Could you check a few things on this model? Use its own coordinates, in mm. Face numbers are marked on the shaded views. Give positions to 0.01 mm unless a question says otherwise; leave off trailing zeros. Order: outer loops, then holes, each group sorted by start corner. A loop starts at its lowest first (then second) coordinate and runs counter-clockwise, first axis right, second up. Notation, with made-up numbers: (81.25, 6) -> (130.25, 6) arc R7 ccw to (130.25, 11) -> close; hole circle Ø6 at (-32, 7). An arc over 180 degrees is marked (long way). Use one line per item in the form item = value. Start each with the question number.
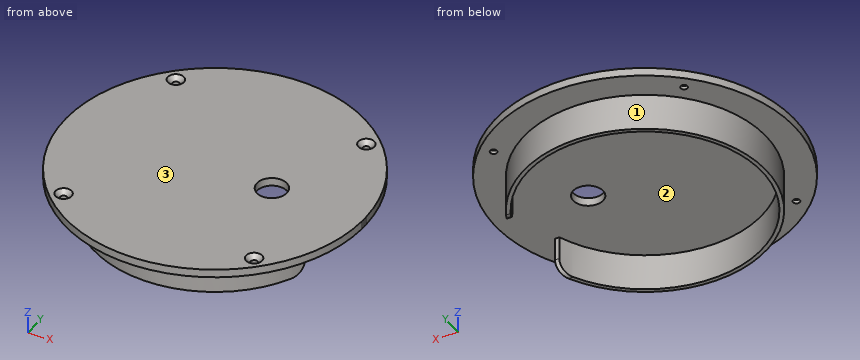
from build123d import *

# Parameters (mm, degrees)
F0_R        = 1.25
F0_R_2      = 5.5
F1_DEPTH    = 3
F3_DEPTH    = 13.4
F4_T1_DEPTH = 26.5968204778
F5_SIZE     = 1.7


# Not quite as in the source:
# - a fillet or chamfer that OpenCascade refuses, or shapes differently, is made with other operations: its cross-section is extruded or revolved along the edge and cut away or added
# - a feature names something its author has since deleted; it is built from what else it names


with BuildPart() as f1:
    # F0 (on Top) → F1 (new body)
    with BuildSketch(Plane.XY):
        with BuildLine():
            ThreePointArc((45.3208194724, 4.0340206186), (-45.5, 0), (45.3208194724, -4.0340206186))
            ThreePointArc((45.3208194724, -4.0340206186), (46.2839051451, -2.086638513), (48.3090053717, -1.3))
            Line((48.3090053717, -1.3), (54.9846342172, -1.3))
            ThreePointArc((54.9846342172, -1.3), (54.9961584201, -0.6500454037), (55, 0))
            ThreePointArc((55, 0), (54.9961584201, 0.6500454037), (54.9846342172, 1.3))
            Line((54.9846342172, 1.3), (48.3090053717, 1.3))
            ThreePointArc((48.3090053717, 1.3), (46.2839051451, 2.086638513), (45.3208194724, 4.0340206186))
        make_face()
        with BuildLine():
            Line((39.2652518138, 1.3), (32, 1.3))
            Line((32, 1.3), (32, 0))
            Line((32, 0), (32, -1.3))
            Line((32, -1.3), (39.2652518138, -1.3))
            ThreePointArc((39.2652518138, -1.3), (41.499054271, -2.2974699547), (42.2474228376, -4.6265822785))
            ThreePointArc((42.2474228376, -4.6265822785), (-42.5, 0), (42.2474228376, 4.6265822785))
            ThreePointArc((42.2474228376, 4.6265822785), (41.499054271, 2.2974699547), (39.2652518138, 1.3))
        make_face(mode=Mode.SUBTRACT)
        with BuildLine():
            Line((32, 15), (32, 1.3))
            Line((32, 1.3), (39.2652518138, 1.3))
            ThreePointArc((39.2652518138, 1.3), (41.499054271, 2.2974699547), (42.2474228376, 4.6265822785))
            ThreePointArc((42.2474228376, 4.6265822785), (-42.5, 0), (42.2474228376, -4.6265822785))
            ThreePointArc((42.2474228376, -4.6265822785), (41.499054271, -2.2974699547), (39.2652518138, -1.3))
            Line((39.2652518138, -1.3), (32, -1.3))
            Line((32, -1.3), (32, -15))
            Line((32, -15), (21.575, -15))
            Line((21.575, -15), (21.575, -17.3))
            ThreePointArc((21.575, -17.3), (17.075, -21.8), (12.575, -17.3))
            Line((12.575, -17.3), (12.575, -15))
            Line((12.575, -15), (-12.575, -15))
            Line((-12.575, -15), (-12.575, -17.3))
            ThreePointArc((-12.575, -17.3), (-17.075, -21.8), (-21.575, -17.3))
            Line((-21.575, -17.3), (-21.575, -15))
            Line((-21.575, -15), (-32, -15))
            Line((-32, -15), (-32, 15))
            Line((-32, 15), (-21.575, 15))
            Line((-21.575, 15), (-21.575, 17.3))
            ThreePointArc((-21.575, 17.3), (-17.075, 21.8), (-12.575, 17.3))
            Line((-12.575, 17.3), (-12.575, 15))
            Line((-12.575, 15), (12.575, 15))
            Line((12.575, 15), (12.575, 17.3))
            ThreePointArc((12.575, 17.3), (17.075, 21.8), (21.575, 17.3))
            Line((21.575, 17.3), (21.575, 15))
            Line((21.575, 15), (32, 15))
        make_face()
        with BuildLine():
            ThreePointArc((48.3090053717, -1.3), (46.2839051451, -2.086638513), (45.3208194724, -4.0340206186))
            ThreePointArc((45.3208194724, -4.0340206186), (-45.5, 0), (45.3208194724, 4.0340206186))
            ThreePointArc((45.3208194724, 4.0340206186), (46.2839051451, 2.086638513), (48.3090053717, 1.3))
            Line((48.3090053717, 1.3), (54.9846342172, 1.3))
            ThreePointArc((54.9846342172, 1.3), (-55, 0), (54.9846342172, -1.3))
            Line((54.9846342172, -1.3), (48.3090053717, -1.3))
        make_face()
        with Locations((-35.175, -35.8856778534)):
            Circle(F0_R, mode=Mode.SUBTRACT)
        with Locations((35.175, -35.8856778534)):
            Circle(F0_R, mode=Mode.SUBTRACT)
        with Locations((-35.175, 35.8856778534)):
            Circle(F0_R, mode=Mode.SUBTRACT)
        with Locations((35.175, 35.8856778534)):
            Circle(F0_R, mode=Mode.SUBTRACT)
        with BuildLine():
            Line((32, 0), (32, 1.3))
            Line((32, 1.3), (32, 15))
            Line((32, 15), (21.575, 15))
            Line((21.575, 15), (21.575, 17.3))
            ThreePointArc((21.575, 17.3), (17.075, 21.8), (12.575, 17.3))
            Line((12.575, 17.3), (12.575, 15))
            Line((12.575, 15), (-12.575, 15))
            Line((-12.575, 15), (-12.575, 17.3))
            ThreePointArc((-12.575, 17.3), (-17.075, 21.8), (-21.575, 17.3))
            Line((-21.575, 17.3), (-21.575, 15))
            Line((-21.575, 15), (-32, 15))
            Line((-32, 15), (-32, -15))
            Line((-32, -15), (-21.575, -15))
            Line((-21.575, -15), (-21.575, -17.3))
            ThreePointArc((-21.575, -17.3), (-17.075, -21.8), (-12.575, -17.3))
            Line((-12.575, -17.3), (-12.575, -15))
            Line((-12.575, -15), (12.575, -15))
            Line((12.575, -15), (12.575, -17.3))
            ThreePointArc((12.575, -17.3), (17.075, -21.8), (21.575, -17.3))
            Line((21.575, -17.3), (21.575, -15))
            Line((21.575, -15), (32, -15))
            Line((32, -15), (32, -1.3))
            Line((32, -1.3), (32, 0))
        make_face()
        with Locations((21, 0)):
            Circle(F0_R_2, mode=Mode.SUBTRACT)
    extrude(amount=F1_DEPTH)

    # F2 (on face) → F3 (join)
    with BuildSketch(Plane(origin=(0, 0, 0), x_dir=(1, 0, 0), z_dir=(0, 0, -1))):
        with BuildLine():
            Line((40.2988833592, 15), (41.895703837, 15))
            ThreePointArc((41.895703837, 15), (-44.5, 0), (41.895703837, -15))
            Line((41.895703837, -15), (40.2988833592, -15))
            ThreePointArc((40.2988833592, -15), (-43, 0), (40.2988833592, 15))
        make_face()
    extrude(amount=F3_DEPTH)

    # F4: fillet of radius 5 on 2 edges, made by hand

    # F4_s2 → F4_t1 (cut)
    with BuildSketch(Plane.YZ.offset(27.7988833592)):
        with BuildLine():
            ThreePointArc((-15, -8.4), (-16.4644660941, -11.9355339059), (-20, -13.4))
            Line((-20, -13.4), (-15, -13.4))
            Line((-15, -13.4), (-15, -8.4))
        make_face()
        with BuildLine():
            ThreePointArc((15, -8.4), (16.4644660941, -11.9355339059), (20, -13.4))
            Line((20, -13.4), (15, -13.4))
            Line((15, -13.4), (15, -8.4))
        make_face()
    extrude(amount=F4_T1_DEPTH, mode=Mode.SUBTRACT)

    # F5
    f5_edges = [f1.edges().sort_by_distance(p)[0] for p in [
        (-36.425, 35.885678, 3),
        (-36.425, -35.885678, 3),
        (33.925, -35.885678, 3),
        (33.925, 35.885678, 3),
    ]]
    chamfer(f5_edges, length=F5_SIZE)


solid = f1.part
(1) Imagine slicing it at A-A (x = 0). Write out the boundary of the cut face in (y, z).
(2) Imagine slicing it at C-C (z = -1.5). Write out the boundary of the cut face in (x, y), plus the area to 3 significant figures.
(3) I'm going to push flat-ended pins straight in: pin 1 Ø1.3 at (x, z) = (41, -3.5) entering from +Y; pin 2 Ø2 at (y, z) = (18, 0.5) entering from +X; pin 3 Ø10 at (x, y) = (21, 0) entering from +Z; pin 4 Ø6 at (x, y) = (-4, -32) entering from -Z. Where does each tip first touch, or does it pass through?
(4) Imagine slicing it at B-B (x = 21). Write out the boundary of the cut face in (y, z), plus the area to 3 significant figures.
(5) Imagine slicing it at D-D (y = 11). Write out the boundary of the cut face in (x, z).
(6) We'd pull the mould along Y, two halves only. Please class the marked faces 1, 2 and 3: pulls with the +Y half, pulls with the -Y half, needs draft (parallel to the pull), parting line crosses it, or undercut.
(7) Please list where these lines run through material, in increasing order: probe 1 along X at (y, z) = (36.5, 0.75); probe 2 along Z at (x, y) = (38, 31); probe 3 along Y at (x, z) = (2, -1.5).
Calculated:
q1.outline = (-55, 0) -> (-44.5, 0) -> (-44.5, -13.4) -> (-43, -13.4) -> (-43, 0) -> (43, 0) -> (43, -13.4) -> (44.5, -13.4) -> (44.5, 0) -> (55, 0) -> (55, 3) -> (-55, 3) -> close
q2.outline = (40.3, -15) arc R43 cw (long way) to (40.3, 15) -> (41.9, 15) arc R44.5 ccw (long way) to (41.9, -15) -> close
q2.area = 366 mm2
q3.pin_1 = 18.77
q3.pin_2 = 52.31
q3.pin_3 = through
q3.pin_4 = 0
q4.outline = (-50.83, 0) -> (-39.23, 0) -> (-39.23, -13.4) -> (-37.52, -13.4) -> (-37.52, 0) -> (-5.5, 0) -> (-5.5, 3) -> (-50.83, 3) -> close; (5.5, 0) -> (37.52, 0) -> (37.52, -13.4) -> (39.23, -13.4) -> (39.23, 0) -> (50.83, 0) -> (50.83, 3) -> (5.5, 3) -> close
q4.area = 318 mm2
q5.outline = (-53.89, 0) -> (-43.12, 0) -> (-43.12, -13.4) -> (-41.57, -13.4) -> (-41.57, 0) -> (53.89, 0) -> (53.89, 3) -> (-53.89, 3) -> close
q6.face_1 = parting line crosses it
q6.face_2 = undercut
q6.face_3 = needs draft
q7.probe_1 = -41.14 to -36.26, -34.09 to 34.09, 36.26 to 41.14
q7.probe_2 = 0 to 3
q7.probe_3 = -44.46 to -42.95, 42.95 to 44.46
